Part model, mm, in its own coordinate system. A direction names the side the tool comes from. Round coordinates to 2 decimals unless told otherwise and drop trailing zeros. Write each loop counter-clockwise with the first axis right and the second up, starting at its lowest first coordinate (ties: lowest second). Pieces come first, ordered by that corner, then holes.
from build123d import *

# Parameters (mm, degrees)
SKETCH1_W           = 10
SKETCH1_H           = 80
BOSS_EXTRUDE1_DEPTH = 5
SKETCH2_R           = 2
BOSS_EXTRUDE2_DEPTH = 5
SKETCH3_W           = 10
SKETCH3_H           = 15
BOSS_EXTRUDE4_DEPTH = 10
FILLET1_R           = 1


with BuildPart() as part:
    # Sketch1 → Boss-Extrude1 (new body)
    with BuildSketch(Plane.XY):
        with Locations((5, 40)):
            Rectangle(SKETCH1_W, SKETCH1_H)
    boss_extrude1 = extrude(amount=BOSS_EXTRUDE1_DEPTH)

    # Sketch2 → Boss-Extrude2 (add)
    with BuildSketch(Plane.XY.offset(5)):
        with Locations(Location((5, 5, 0), (0, 0, 180))):
            Circle(SKETCH2_R)
        with Locations(Location((5, 34.285714286, 0), (0, 0, 180))):
            Circle(SKETCH2_R)
    boss_extrude2 = extrude(amount=BOSS_EXTRUDE2_DEPTH)

    # Mirror2: Boss-Extrude1, Boss-Extrude2 across plane
    add(boss_extrude1.mirror(Plane(origin=(5, 34.285714286, 10), x_dir=(1, 0, 0), z_dir=(0, 0, 1))))
    add(boss_extrude2.mirror(Plane(origin=(5, 34.285714286, 10), x_dir=(1, 0, 0), z_dir=(0, 0, 1))))

    # Sketch3 → Boss-Extrude4 (add)
    with BuildSketch(Plane.XY.offset(5)):
        with Locations((5, 72.5)):
            Rectangle(SKETCH3_W, SKETCH3_H)
    extrude(amount=BOSS_EXTRUDE4_DEPTH)

    # Fillet1
    fillet1_edges = [part.edges().sort_by_distance(p)[0] for p in [
        (0, 40, 20),
        (5, 0, 20),
        (10, 40, 20),
        (5, 80, 20),
        (5, 80, 0),
        (10, 40, 0),
        (5, 0, 0),
        (0, 40, 0),
        (0, 80, 10),
        (10, 80, 10),
    ]]
    fillet(fillet1_edges, radius=FILLET1_R)


solid = part.part
Q1. Saw through at C-C, the plane x = 2. Write the cut outline in (y, z).
Q2. Two-plate mould, pull along Z, no slides. Class faces 4 (the flat face through (7, 33, 15)), 5 (the flat face through (5, 0, 17)), 6 (the flat face through (5, 41, 20)): released by +Z, released by -Z, zero draft, split by the parting line, or undercut.
Q3. Wall check: line 1 (Z direction, x = 7, y = 33); line 2 (Y direction, x = 6.5, z = 10.75); line 3 (Z direction, x = 9.5, y = 62.5). Give the ranges that are in metal, low to high.
Q4. Tool access for faces 1 (the flat face through (5, 65, 10)), 2 (the flat face through (0, 48, 16)), 3 (the cylindrical face through (6.6, 6.2, 9.9)): list every direction of +Z, -Z, +X, -X, +Y, -Y with a clear straight run to the whole face (end or side of a thin tool).
Q5. Drop a flat-ended pin along its axis: P1, Ø4, axis at y = 62, z = 8, coming from the -X side. Give the stop position or say it passes through.
Q6. Saw through at B-B, the plane x = 5. Write the cut outline in (y, z).
Q7. Saw through at D-D, the plane z = 11. Write the cut outline in (x, y), and give its area (3 significant figures).
Q8. Saw through at A-A, the plane y = 11.5. Write the cut outline in (x, z).
Computed:
1. outline: (0, 1) arc R1 ccw to (1, 0) - (79, 0) arc R1 ccw to (80, 1) - (80, 19) arc R1 ccw to (79, 20) - (1, 20) arc R1 ccw to (0, 19) - (0, 15) - (65, 15) - (65, 5) - (0, 5) - close
2. face 4: undercut
2. face 5: zero draft
2. face 6: released by +Z
3. line 1: z = 0 to 5, 15 to 20
3. line 2: y = 3.68 to 6.32, 32.96 to 35.61, 65 to 80
3. line 3: z = 0.13 to 5, 15 to 19.87
4. face 1: +X, -X
4. face 2: +Z, -Z, -X, +Y, -Y
4. face 3: none
5. P1: passes through
6. outline: (0, 1) arc R1 ccw to (1, 0) - (79, 0) arc R1 ccw to (80, 1) - (80, 19) arc R1 ccw to (79, 20) - (1, 20) arc R1 ccw to (0, 19) - (0, 15) - (3, 15) - (3, 5) - (0, 5) - close; hole (7, 5) - (32.29, 5) - (32.29, 15) - (7, 15) - close; hole (36.29, 5) - (65, 5) - (65, 15) - (36.29, 15) - close
7. outline: (0, 65) - (10, 65) - (10, 79) arc R1 ccw to (9, 80) - (1, 80) arc R1 ccw to (0, 79) - close; circle Ø4 at (5, 5); circle Ø4 at (5, 34.29)
7. area: 175 mm2
8. outline: (0, 1) arc R1 ccw to (1, 0) - (9, 0) arc R1 ccw to (10, 1) - (10, 5) - (0, 5) - close; (0, 15) - (10, 15) - (10, 19) arc R1 ccw to (9, 20) - (1, 20) arc R1 ccw to (0, 19) - close
